from build123d import *

# Parameters (mm, degrees)
SKETCH1_R           = 2.356484411
SKETCH1_R_2         = 3.356538595
SKETCH1_R_3         = 3.175
SKETCH1_R_4         = 4.064709562
SKETCH1_R_5         = 2.555437721
SKETCH1_R_6         = 3.242334338
SKETCH1_R_7         = 2.462755239
BOSS_EXTRUDE1_DEPTH = 38.1


with BuildPart() as part:
    # Sketch1 → Boss-Extrude1 (new body)
    with BuildSketch(Plane(origin=(0, 0, 0), x_dir=(1, 0, 0), z_dir=(0, 1, 0))):
        with BuildLine():
            Line((-74.6125, 15.473036022), (-74.6125, -15.473036022))
            ThreePointArc((-74.6125, -15.473036022), (-52.874683743, -54.86991725), (-12.7, -75.134213245))
            Line((-12.7, -75.134213245), (12.7, -75.134213245))
            ThreePointArc((12.7, -75.134213245), (52.874683743, -54.86991725), (74.6125, -15.473036022))
            Line((74.6125, -15.473036022), (74.6125, 15.473036022))
            ThreePointArc((74.6125, 15.473036022), (66.568680107, 37.081677804), (52.429845716, 55.295128883))
            Line((52.429845716, 55.295128883), (23.6855, 82.55))
            Line((23.6855, 82.55), (19.05, 82.55))
            Line((19.05, 82.55), (19.05, 76.2))
            Line((19.05, 76.2), (0, 76.2))
            ThreePointArc((0, 76.2), (-1.309576606, 76.036760248), (-2.539006662, 75.557031324))
            Line((-2.539006662, 75.557031324), (-55.150410299, 47.084918442))
            ThreePointArc((-55.150410299, 47.084918442), (-63.168001103, 40.936392006), (-68.874977996, 32.598733198))
            ThreePointArc((-68.874977996, 32.598733198), (-72.252933929, 24.206477205), (-74.6125, 15.473036022))
        make_face()
        with Locations((23.6855, 74.812542953)):
            Circle(SKETCH1_R, mode=Mode.SUBTRACT)
        with Locations((-25.953983408, 25.159074147)):
            Circle(SKETCH1_R_2, mode=Mode.SUBTRACT)
        with Locations((-41.987680119, 28.850105121)):
            Circle(SKETCH1_R_3, mode=Mode.SUBTRACT)
        with Locations((41.987680119, 28.850105121)):
            Circle(SKETCH1_R_3, mode=Mode.SUBTRACT)
        with Locations((-41.987680119, -28.850105121)):
            Circle(SKETCH1_R_3, mode=Mode.SUBTRACT)
        with Locations((41.987680119, -28.850105121)):
            Circle(SKETCH1_R_3, mode=Mode.SUBTRACT)
        with Locations((-33.451838253, 28.850105121)):
            Circle(SKETCH1_R_3, mode=Mode.SUBTRACT)
        with Locations((33.451838253, 28.850105121)):
            Circle(SKETCH1_R_3, mode=Mode.SUBTRACT)
        with Locations((-33.451838253, -28.850105121)):
            Circle(SKETCH1_R_3, mode=Mode.SUBTRACT)
        with Locations((33.451838253, -28.850105121)):
            Circle(SKETCH1_R_3, mode=Mode.SUBTRACT)
        with Locations((-58.499626731, 35.97459363)):
            Circle(SKETCH1_R_4, mode=Mode.SUBTRACT)
        with Locations((60.460006294, 34.52310187)):
            Circle(SKETCH1_R_5, mode=Mode.SUBTRACT)
        with Locations((-58.499626731, -35.97459363)):
            Circle(SKETCH1_R_4, mode=Mode.SUBTRACT)
        with Locations((61.236723994, -34.882223147)):
            Circle(SKETCH1_R_6, mode=Mode.SUBTRACT)
        with Locations((25.953983408, 25.159074147)):
            Circle(SKETCH1_R_2, mode=Mode.SUBTRACT)
        with Locations((25.953983408, -25.159074147)):
            Circle(SKETCH1_R_2, mode=Mode.SUBTRACT)
        with Locations((-25.953983408, -25.159074147)):
            Circle(SKETCH1_R_2, mode=Mode.SUBTRACT)
        with Locations((70.02564652, 8.562540674)):
            Circle(SKETCH1_R_7, mode=Mode.SUBTRACT)
        with Locations((-70.02564652, 8.562540674)):
            Circle(SKETCH1_R_7, mode=Mode.SUBTRACT)
        with Locations((70.02564652, -8.562540674)):
            Circle(SKETCH1_R_7, mode=Mode.SUBTRACT)
        with Locations((-70.02564652, -8.562540674)):
            Circle(SKETCH1_R_7, mode=Mode.SUBTRACT)
        with Locations((-70.02564652, 0)):
            Circle(SKETCH1_R_7, mode=Mode.SUBTRACT)
        with Locations((70.02564652, 0)):
            Circle(SKETCH1_R_7, mode=Mode.SUBTRACT)
        Polygon((20.955, 37.465), (-20.955, 37.465), (-20.955, 0), (-20.955, -37.465), (20.955, -37.465), (20.955, 0), align=None, mode=Mode.SUBTRACT)
        with BuildLine():
            Line((-53.975, 19.3675), (-50.4825, 19.3675))
            Line((-50.4825, 19.3675), (-46.99, 22.86))
            Line((-46.99, 22.86), (-33.451838253, 22.86))
            ThreePointArc((-33.451838253, 22.86), (-31.838145049, 22.596886364), (-30.391611171, 21.834800884))
            Line((-30.391611171, 21.834800884), (-27.038772918, 19.304356919))
            ThreePointArc((-27.038772918, 19.304356919), (-25.551893581, 17.514555641), (-25.019, 15.249556036))
            Line((-25.019, 15.249556036), (-25.019, 0))
            Line((-25.019, 0), (-25.019, -15.249556036))
            ThreePointArc((-25.019, -15.249556036), (-25.551893581, -17.514555641), (-27.038772918, -19.304356919))
            Line((-27.038772918, -19.304356919), (-30.391611171, -21.834800884))
            ThreePointArc((-30.391611171, -21.834800884), (-31.838145049, -22.596886364), (-33.451838253, -22.86))
            Line((-33.451838253, -22.86), (-46.99, -22.86))
            Line((-46.99, -22.86), (-50.4825, -19.3675))
            Line((-50.4825, -19.3675), (-53.975, -19.3675))
            ThreePointArc((-53.975, -19.3675), (-54.873025612, -19.739474388), (-55.245, -20.6375))
            Line((-55.245, -20.6375), (-55.245, -27.305))
            ThreePointArc((-55.245, -27.305), (-55.616974388, -28.203025612), (-56.515, -28.575))
            Line((-56.515, -28.575), (-63.5, -28.575))
            ThreePointArc((-63.5, -28.575), (-64.398025612, -28.203025612), (-64.77, -27.305))
            Line((-64.77, -27.305), (-64.77, 27.305))
            ThreePointArc((-64.77, 27.305), (-64.398025612, 28.203025612), (-63.5, 28.575))
            Line((-63.5, 28.575), (-56.515, 28.575))
            ThreePointArc((-56.515, 28.575), (-55.616974388, 28.203025612), (-55.245, 27.305))
            Line((-55.245, 27.305), (-55.245, 20.6375))
            ThreePointArc((-55.245, 20.6375), (-54.873025612, 19.739474388), (-53.975, 19.3675))
        make_face(mode=Mode.SUBTRACT)
        with BuildLine():
            Line((64.77, 27.305), (64.77, -27.305))
            ThreePointArc((64.77, -27.305), (64.398025612, -28.203025612), (63.5, -28.575))
            Line((63.5, -28.575), (56.515, -28.575))
            ThreePointArc((56.515, -28.575), (55.616974388, -28.203025612), (55.245, -27.305))
            Line((55.245, -27.305), (55.245, -20.6375))
            ThreePointArc((55.245, -20.6375), (54.873025612, -19.739474388), (53.975, -19.3675))
            Line((53.975, -19.3675), (50.4825, -19.3675))
            Line((50.4825, -19.3675), (46.99, -22.86))
            Line((46.99, -22.86), (33.451838253, -22.86))
            ThreePointArc((33.451838253, -22.86), (31.838145049, -22.596886364), (30.391611171, -21.834800884))
            Line((30.391611171, -21.834800884), (27.038772918, -19.304356919))
            ThreePointArc((27.038772918, -19.304356919), (25.551893581, -17.514555641), (25.019, -15.249556036))
            Line((25.019, -15.249556036), (25.019, 0))
            Line((25.019, 0), (25.019, 15.249556036))
            ThreePointArc((25.019, 15.249556036), (25.551893581, 17.514555641), (27.038772918, 19.304356919))
            Line((27.038772918, 19.304356919), (30.391611171, 21.834800884))
            ThreePointArc((30.391611171, 21.834800884), (31.838145049, 22.596886364), (33.451838253, 22.86))
            Line((33.451838253, 22.86), (46.99, 22.86))
            Line((46.99, 22.86), (50.4825, 19.3675))
            Line((50.4825, 19.3675), (53.975, 19.3675))
            ThreePointArc((53.975, 19.3675), (54.873025612, 19.739474388), (55.245, 20.6375))
            Line((55.245, 20.6375), (55.245, 27.305))
            ThreePointArc((55.245, 27.305), (55.616974388, 28.203025612), (56.515, 28.575))
            Line((56.515, 28.575), (63.5, 28.575))
            ThreePointArc((63.5, 28.575), (64.398025612, 28.203025612), (64.77, 27.305))
        make_face(mode=Mode.SUBTRACT)
        with BuildLine():
            Line((-20.845950883, 41.338131188), (0, 41.338131188))
            Line((0, 41.338131188), (20.900876069, 41.338131188))
            ThreePointArc((20.900876069, 41.338131188), (23.189592711, 40.793346302), (24.987420284, 39.275838327))
            Line((24.987420284, 39.275838327), (27.196988383, 36.283666683))
            ThreePointArc((27.196988383, 36.283666683), (28.994815956, 34.766158708), (31.283532598, 34.221373822))
            Line((31.283532598, 34.221373822), (50.45628088, 34.221373822))
            ThreePointArc((50.45628088, 34.221373822), (55.31708187, 37.516208085), (54.056832983, 43.251632379))
            Line((54.056832983, 43.251632379), (32.348707377, 63.834886263))
            ThreePointArc((32.348707377, 63.834886263), (25.730530949, 68.068574663), (18.014985698, 69.550039535))
            Line((18.014985698, 69.550039535), (1.55163213, 69.550039535))
            ThreePointArc((1.55163213, 69.550039535), (-5.413950327, 68.681774216), (-11.953236682, 66.130116403))
            Line((-11.953236682, 66.130116403), (-49.707341043, 45.69844101))
            ThreePointArc((-49.707341043, 45.69844101), (-52.830230484, 39.073656263), (-47.091531492, 34.52310187))
            Line((-47.091531492, 34.52310187), (-31.086999544, 34.52310187))
            ThreePointArc((-31.086999544, 34.52310187), (-28.840846685, 35.046656179), (-27.057679262, 36.509402133))
            Line((-27.057679262, 36.509402133), (-24.875271165, 39.351830925))
            ThreePointArc((-24.875271165, 39.351830925), (-23.092103742, 40.814576878), (-20.845950883, 41.338131188))
        make_face(mode=Mode.SUBTRACT)
        with BuildLine():
            Line((-23.854336738, -60.495536567), (0, -60.495536567))
            Line((0, -60.495536567), (12.7, -67.96894498))
            ThreePointArc((12.7, -67.96894498), (38.322472705, -59.497281046), (58.80689112, -41.928308409))
            Line((58.80689112, -41.928308409), (54.275996481, -36.293661738))
            ThreePointArc((54.275996481, -36.293661738), (53.394000982, -35.594661364), (52.296567671, -35.345346879))
            Line((52.296567671, -35.345346879), (33.457769344, -35.345346879))
            ThreePointArc((33.457769344, -35.345346879), (32.159314658, -35.702317921), (31.225829045, -36.672893786))
            Line((31.225829045, -36.672893786), (29.270713217, -40.271962344))
            ThreePointArc((29.270713217, -40.271962344), (28.337227604, -41.242538208), (27.038772918, -41.599509251))
            Line((27.038772918, -41.599509251), (-27.038772918, -41.599509251))
            ThreePointArc((-27.038772918, -41.599509251), (-28.216614381, -41.30990688), (-29.125868694, -40.507138769))
            Line((-29.125868694, -40.507138769), (-32.269685191, -35.97459363))
            ThreePointArc((-32.269685191, -35.97459363), (-33.178939505, -35.171825519), (-34.356780968, -34.882223147))
            Line((-34.356780968, -34.882223147), (-44.859278162, -34.882223147))
            ThreePointArc((-44.859278162, -34.882223147), (-46.655329386, -35.626171923), (-47.399278162, -37.422223147))
            Line((-47.399278162, -37.422223147), (-47.399278162, -46.454771748))
            ThreePointArc((-47.399278162, -46.454771748), (-36.419314032, -54.804107481), (-23.854336738, -60.495536567))
        make_face(mode=Mode.SUBTRACT)
    extrude(amount=BOSS_EXTRUDE1_DEPTH)


solid = part.part
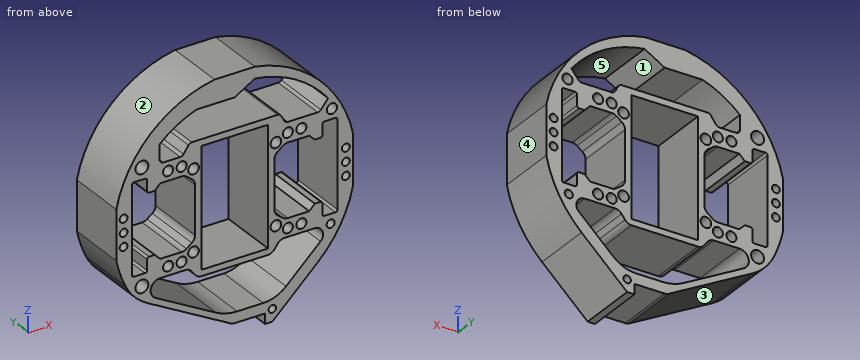
Design review of the part built by this model. Coordinates are the model's own, in mm. Face numbers are marked on the shaded views. A direction names the side the tool comes from. Coordinates: 2 decimals unless noted, no trailing zeros. Order: outer loops, then holes, each group sorted by start corner. A loop starts at its lowest first (then second) coordinate and runs counter-clockwise, first axis right, second up. Notation, with made-up numbers: (74.25, 76) -> (126.25, 76) arc R29 cw to (126.25, 104) -> close; hole circle Ø11 at (53.5, -13.75). An arc over 180 degrees is marked (long way). Use one line per item in the form item = value. Start each with the question number.
(1) For the marked faces 4 and 5, list the 3-axis set-ups (+Z, -Z, +X, -X, +Y, -Y) from which the entire face can be reached by the end or side of a thin tool; tool diameter is ignored.
(2) Add section A-A on z = 0. State the section outline as (x, y) points (1 decimal).
(3) Insertion check: pin 1 (2 mm diameter, centred on x = 35.5, y = 26.5, fed in from -Z); pin 2 (9.5 mm diameter, centred on x = 8.5, y = 15, fed in from -Z); pin 3 (8.5 mm diameter, centred on x = 25.95, z = -25.16, fed in from -Y); pin 4 (7 mm diameter, centred on x = 38, y = 13.5, fed in from +Z). Each pin has a flat end and moves straight along its axis. Give the tip position at first contact, or say it passes through.
(4) The part is to be moulded in two halves that separate along Z. For the marked faces 1, 2 and 3, say which applies: +Z half, -Z half, draft (parallel to the pull), parting line (faces both ways), or undercut.
(5) For probe 1 along X at (y, z) = (33, 5) (1 decimal); probe 2 along X at (y, z) = (17, 0) (1 decimal); probe 3 along Z at (x, y) = (49, 16.5), list the stretches that pass through material, from the lowest coordinate up.
(6) Add section B-B on z = 55. State the section outline as (x, y) points.
(7) Add section C-C on y = 14.5. Give the number of separate pieces and of enclosed holes in the cut face, plus the area to 3 significant figures.
Answer block:
q1.face_4 = +Z, -Z, +X, +Y, -Y
q1.face_5 = +Y, -Y
q2.outline = (-74.6, 0) -> (-72.5, 0) -> (-72.5, 38.1) -> (-74.6, 38.1) -> close; (-67.6, 0) -> (-64.8, 0) -> (-64.8, 38.1) -> (-67.6, 38.1) -> close; (-25, 0) -> (-21, 0) -> (-21, 38.1) -> (-25, 38.1) -> close; (21, 0) -> (25, 0) -> (25, 38.1) -> (21, 38.1) -> close; (64.8, 0) -> (67.6, 0) -> (67.6, 38.1) -> (64.8, 38.1) -> close; (72.5, 0) -> (74.6, 0) -> (74.6, 38.1) -> (72.5, 38.1) -> close
q3.pin_1 = -72.3
q3.pin_2 = -76.2
q3.pin_3 = 0
q3.pin_4 = 67.94
q4.face_1 = undercut
q4.face_2 = +Z half
q4.face_3 = -Z half
q5.probe_1 = -74.6 to -64.8, -25 to -21, 21 to 25, 64.8 to 74.6
q5.probe_2 = -74.6 to -72.5, -67.6 to -64.8, -25 to -21, 21 to 25, 64.8 to 67.6, 72.5 to 74.6
q5.probe_3 = -58.55 to -48.05, -34.22 to -20.85, 20.85 to 35.35, 52.07 to 58.36
q6.outline = (-52.74, 0) -> (-36.09, 0) -> (-36.09, 38.1) -> (-52.74, 38.1) -> close; (45.28, 0) -> (52.74, 0) -> (52.74, 38.1) -> (45.28, 38.1) -> close
q7.separate_pieces = 1
q7.enclosed_holes = 28
q7.area = 5,860 mm²
